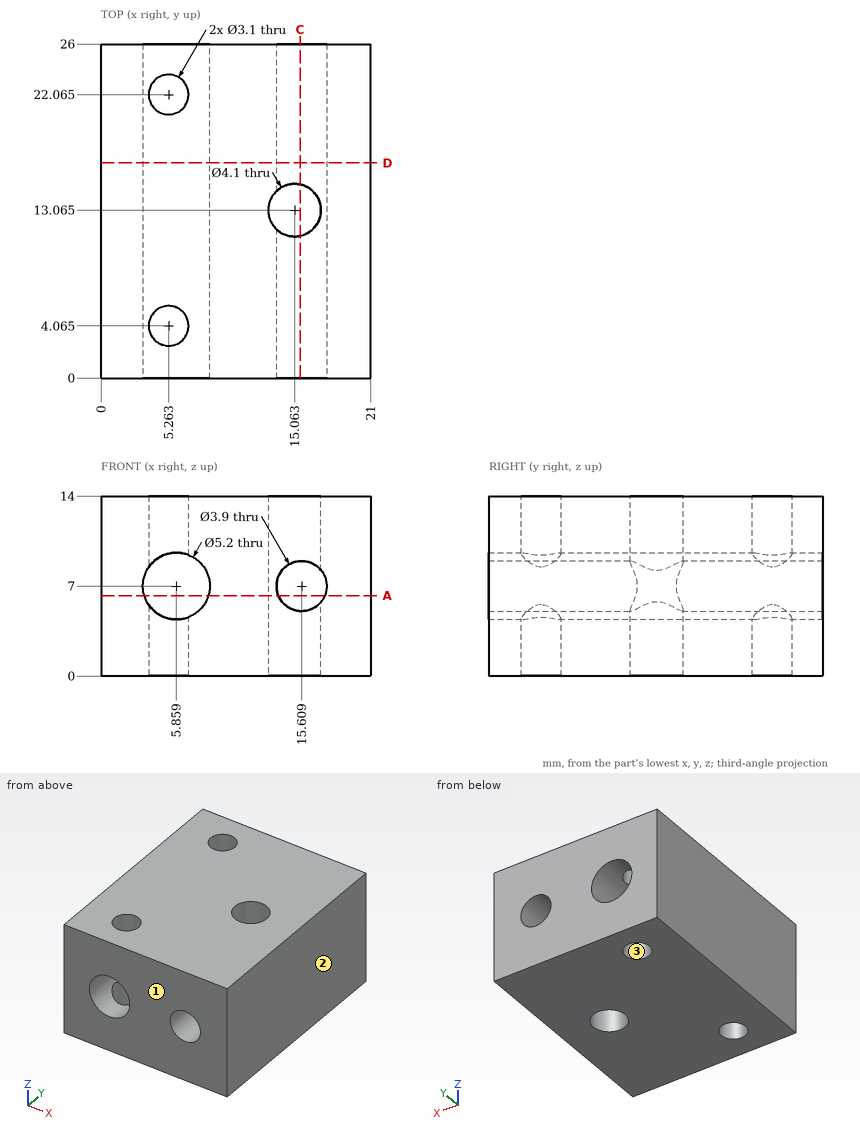
Verification items for this drawing (mm, ordinates from the low corner). Coordinates: 2 decimals unless noted, no trailing zeros. Write each loop counter-clockwise with the first axis right and the second up, starting at its lowest first coordinate (ties: lowest second). Pieces come first, ordered by that corner, then holes. Notation, with made-up numbers: (33.5, 50.5) - (39.5, 50.5) arc R18 cw to (39.5, 77.5) - close; hole circle Ø8 at (37, 3). An arc over 180 degrees is marked (long way). One line per question, with ' | ' between items.
Item 1: Sectioned sample at D-D on y = 16.75. Record the boundary of the cut face in (x, z).
Determined:
outline: (0, 0) - (21, 0) - (21, 14) - (0, 14) - close; hole circle Ø5.2 at (5.86, 7); hole circle Ø3.9 at (15.61, 7)
Item 2: Gauge pin test, flat end, axial feed: P1, Ø1.9, axis at x = 5.26, y = 4.07, coming from the -Z side. Record the tip position at first contact, or that the pin passes through.
Determined:
P1: passes through
Item 3: Mould release check, pull along X, two halves, no side actions. Record for the marked faces 1, 2 and 3: pulls with the +X half, pulls with the -X half, needs draft (parallel to the pull), parting line crosses it, or undercut.
Determined:
face 1: needs draft | face 2: pulls with the +X half | face 3: undercut
Item 4: Sectioned sample at C-C on x = 15.5. Record the boundary of the cut face in (y, z).
Determined:
outline: (0, 0) - (11.06, 0) - (11.06, 5.05) - (0, 5.05) - close; (0, 8.95) - (11.06, 8.95) - (11.06, 14) - (0, 14) - close; (15.07, 0) - (26, 0) - (26, 5.05) - (15.07, 5.05) - close; (15.07, 8.95) - (26, 8.95) - (26, 14) - (15.07, 14) - close
Item 5: Thickness scan on line 1 (Y direction, x = 5.25, z = 4) (1 decimal); line 2 (X direction, y = 13, z = 9.75); line 3 (X direction, y = 18.5, z = 7.75). Record the ranges inside material, lowest first. Write a range as [from, to].
Determined:
line 1: y = [0, 2.5], [5.6, 20.5], [23.6, 26] | line 2: x = [0, 13.01], [17.11, 21] | line 3: x = [0, 3.37], [8.35, 13.81], [17.41, 21]
Item 6: Sectioned sample at A-A on z = 6.25. Give the number of separate pieces and of enclosed holes in the cut face, plus the area to 3 significant figures.
Determined:
separate pieces: 3 | enclosed holes: 0 | area: 321 mm2
